Geometry: see drawing. Coordinates: mm, zero at the bounding-box minimum. A direction names the side the tool comes from. Coordinates: 2 decimals unless noted, no trailing zeros. Order: outer loops, then holes, each group sorted by start corner. A loop starts at its lowest first (then second) coordinate and runs counter-clockwise, first axis right, second up. Notation, with made-up numbers: M 77,27.25 L 89,27.25 A14 cw 89,42.25 Z; hole C 86.5,85 d10. An arc over 180 degrees is marked long. Answer in a Markdown table with one row per item.
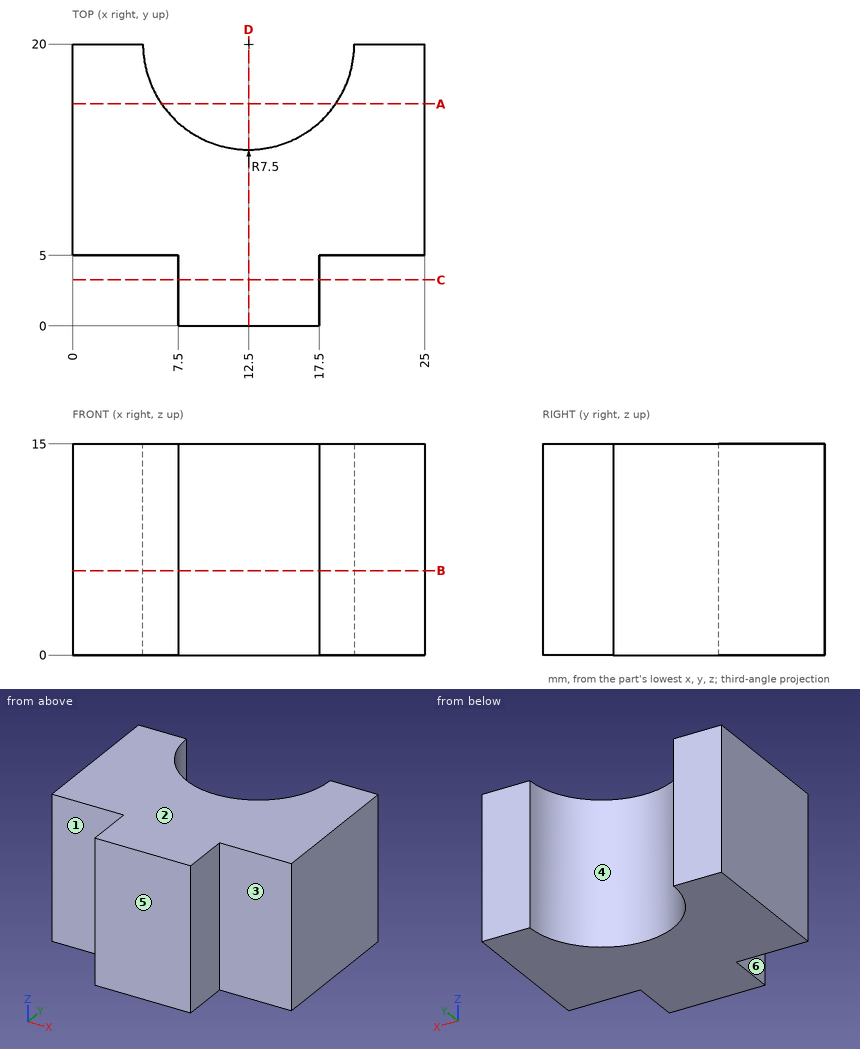
1) Material intervals for probe 1 along Y at (x, z) = (1.5, 10); probe 2 along X at (y, z) = (3, 11.75); probe 3 along X at (y, z) = (17.5, 13.5), sorted ascending.
Resolved:
| item | result |
|---|---|
| probe 1 | y = 5 to 20 |
| probe 2 | x = 7.5 to 17.5 |
| probe 3 | x = 0 to 5.43, 19.57 to 25 |
2) Cut plane D-D, the plane x = 12.5. Output: boundary loops of the cut face in (y, z).
Resolved:
| item | result |
|---|---|
| outline | M 0,0 L 12.5,0 L 12.5,15 L 0,15 Z |
3) Contact query for flat-ended pins moving along their axis: pin 1 (4 mm diameter, centred on y = 14, z = 9.5, fed in from -X); pin 2 (2 mm diameter, centred on x = 3.5, z = 7.5, fed in from -Y); pin 3 (1.5 mm diameter, centred on y = 3, z = 9, fed in from +X). Output: stop coordinate, or through.
Resolved:
| item | result |
|---|---|
| pin 1 | stops at x = 0 |
| pin 2 | stops at y = 5 |
| pin 3 | stops at x = 17.5 |
4) Cut plane B-B, the plane z = 6. Output: boundary loops of the cut face in (x, y), and give its area (3 significant figures).
Resolved:
| item | result |
|---|---|
| outline | M 0,5 L 7.5,5 L 7.5,0 L 17.5,0 L 17.5,5 L 25,5 L 25,20 L 20,20 A7.5 cw 5,20 L 0,20 Z |
| area | 337 mm2 |
5) Mould query, pull axis X, two halves, no side actions, for the marked faces 4, 5 and 6. Classes: +X half, -X half, draft (parallel to the pull), parting line (faces both ways), or undercut.
Resolved:
| item | result |
|---|---|
| face 4 | undercut |
| face 5 | draft |
| face 6 | -X half |
6) Cut plane C-C, the plane y = 3.25. Output: boundary loops of the cut face in (x, z), and give its area (3 significant figures).
Resolved:
| item | result |
|---|---|
| outline | M 7.5,0 L 17.5,0 L 17.5,15 L 7.5,15 Z |
| area | 150 mm2 |
7) Reachability of the marked faces 1, 2 and 3 from +Z, -Z, +X, -X, +Y, -Y: full face, straight path, thin tool, end or side. Return the list, or none.
Resolved:
| item | result |
|---|---|
| face 1 | +Z, -Z, -X, -Y |
| face 2 | +Z, +X, -X, +Y, -Y |
| face 3 | +Z, -Z, +X, -Y |
8) Cut plane A-A, the plane y = 15.75. Output: boundary loops of the cut face in (x, z), and give its area (3 significant figures).
Resolved:
| item | result |
|---|---|
| outline | M 0,0 L 6.32,0 L 6.32,15 L 0,15 Z; M 18.68,0 L 25,0 L 25,15 L 18.68,15 Z |
| area | 190 mm2 |
